The listing builds one solid part. Answer for the finished solid, in the listing's coordinates (mm). Round coordinates to 2 decimals unless told otherwise and drop trailing zeros. Write each loop counter-clockwise with the first axis right and the second up, starting at its lowest first coordinate (ties: lowest second). Pieces come first, ordered by that corner, then holes.
(1) A cutting plane is placed at A-A, the plane z = 261. Give the vertices of the cut face in (x, y), and give its area (3 significant figures).
(2) A cutting plane is placed at B-B, the plane x = 0. Give the number of separate pieces and of enclosed holes in the cut face, and give its area (3 significant figures).
(3) This flat-tipped pin is pushed along its axis until it touches: pin 1 Ø2.5 at (y, z) = (-9, 447.5) entering from -X. Where does it stop, or does it pass through?
(4) Find the intervals of material crossed by probe 1 along Y at (x, z) = (-0.25, 284); probe 2 along Y at (x, z) = (4.7, 47.5); probe 3 along X at (y, z) = (17, 211), in increasing order.
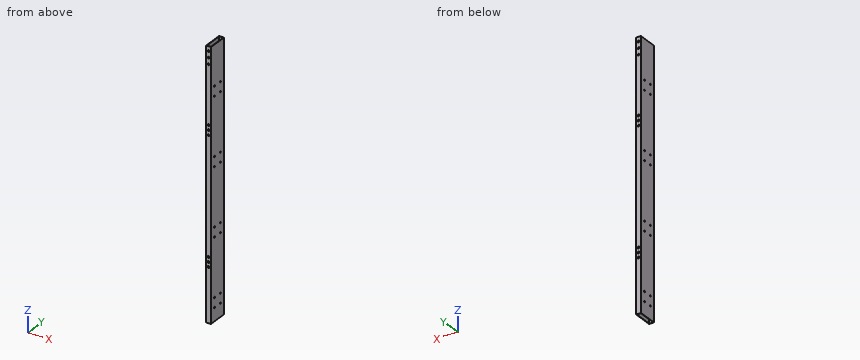
from build123d import *

# Parameters (mm, degrees)
SKETCH_1_W         = 10
SKETCH_1_H         = 40
SKETCH_1_W_2       = 8
SKETCH_1_H_2       = 38
EXTRUDE_1_DEPTH    = 550
SKETCH1_R          = 1.5
CUT_EXTRUDE1_DEPTH = 10
LPATTERN1_COUNT    = 4
LPATTERN1_PITCH    = 140
SKETCH2_R          = 2
CUT_EXTRUDE2_DEPTH = 40
SKETCH3_R          = 2
CUT_EXTRUDE3_DEPTH = 40


with BuildPart() as part:
    # 草图1 → 凸台-拉伸1 (new body)
    with BuildSketch(Plane.XY):
        Rectangle(SKETCH_1_W, SKETCH_1_H)
        Rectangle(SKETCH_1_W_2, SKETCH_1_H_2, mode=Mode.SUBTRACT)
    extrude(amount=EXTRUDE_1_DEPTH)

    # Sketch1 → Cut-Extrude1 (cut)
    with BuildSketch(Plane(origin=(5, 0, 0), x_dir=(0, 0, -1), z_dir=(1, 0, 0))):
        with Locations((-27.5, 9)):
            Circle(SKETCH1_R)
        with Locations((-47.5, 9)):
            Circle(SKETCH1_R)
        with Locations((-27.5, -9)):
            Circle(SKETCH1_R)
        with Locations((-47.5, -9)):
            Circle(SKETCH1_R)
    cut_extrude1 = extrude(amount=-CUT_EXTRUDE1_DEPTH, mode=Mode.SUBTRACT)

    # LPattern1: Cut-Extrude1 ×4
    with Locations(*[(0, 0, i * LPATTERN1_PITCH) for i in range(1, LPATTERN1_COUNT)]):
        add(cut_extrude1, mode=Mode.SUBTRACT)

    # Sketch2 → Cut-Extrude2 (cut)
    with BuildSketch(Plane(origin=(0, 20, 0), x_dir=(1, 0, 0), z_dir=(0, 1, 0))):
        with Locations(Location((0, -111.5, 0), (0, 0, 270))):
            Circle(SKETCH2_R)
        with Locations(Location((0, -121.5, 0), (0, 0, 270))):
            Circle(SKETCH2_R)
        with Locations(Location((0, -131.5, 0), (0, 0, 270))):
            Circle(SKETCH2_R)
        with Locations(Location((0, -373.5, 0), (0, 0, 270))):
            Circle(SKETCH2_R)
        with Locations(Location((0, -383.5, 0), (0, 0, 270))):
            Circle(SKETCH2_R)
        with Locations(Location((0, -393.5, 0), (0, 0, 270))):
            Circle(SKETCH2_R)
    extrude(amount=-CUT_EXTRUDE2_DEPTH, mode=Mode.SUBTRACT)

    # Sketch3 → Cut-Extrude3 (cut)
    with BuildSketch(Plane(origin=(0, 20, 0), x_dir=(1, 0, 0), z_dir=(0, 1, 0))):
        with Locations(Location((0, -540.5, 0), (0, 0, 270))):
            Circle(SKETCH3_R)
        with Locations(Location((0, -527.5, 0), (0, 0, 270))):
            Circle(SKETCH3_R)
        with Locations(Location((0, -514.5, 0), (0, 0, 270))):
            Circle(SKETCH3_R)
    extrude(amount=-CUT_EXTRUDE3_DEPTH, mode=Mode.SUBTRACT)


solid = part.part
Solutions:
1. outline: (-5, -20) - (5, -20) - (5, 20) - (-5, 20) - close; hole (-4, -19) - (4, -19) - (4, 19) - (-4, 19) - close
1. area: 96.0 mm2
2. separate pieces: 20
2. enclosed holes: 0
2. area: 1,030 mm2
3. pin 1: passes through
4. probe 1: y = -20 to -19, 19 to 20
4. probe 2: y = -20 to -10.5, -7.5 to 7.5, 10.5 to 20
4. probe 3: x = -5 to -4, 4 to 5
